```python
from build123d import *

# Parameters (mm, degrees)
SKETCH_1_W      = 35
SKETCH_1_H      = 80
EXTRUDE_1_DEPTH = 5
SKETCH_2_W      = 35
SKETCH_2_H      = 5
SKETCH_2_W_2    = 30
SKETCH_2_W_3    = 5
SKETCH_2_H_2    = 30
EXTRUDE_2_DEPTH = 45
FILLET_2_R      = 3


with BuildPart() as part:
    # 草圖1 → 填料-伸長1 (new body)
    with BuildSketch(Plane.XY):
        with Locations((-29.638177138, -5.194805195)):
            Rectangle(SKETCH_1_W, SKETCH_1_H)
    extrude(amount=EXTRUDE_1_DEPTH)

    # 草圖2 → 填料-伸長2 (add)
    with BuildSketch(Plane.XY.offset(5)):
        with Locations((-29.638177138, 32.305194805)):
            Rectangle(SKETCH_2_W, SKETCH_2_H)
        with Locations((-32.138177138, -42.694805195)):
            Rectangle(SKETCH_2_W_2, SKETCH_2_H)
        with Locations((-14.638177138, -42.694805195)):
            Rectangle(SKETCH_2_W_3, SKETCH_2_H)
        with Locations((-14.638177138, -25.194805195)):
            Rectangle(SKETCH_2_W_3, SKETCH_2_H_2)
    extrude(amount=EXTRUDE_2_DEPTH)

    # 圓角2
    fillet_2_edges = [part.edges().sort_by_distance(p)[0] for p in [
        (-47.138177138, -42.694805195, 50),
        (-14.638177138, -10.194805195, 50),
        (-47.138177138, 32.305194805, 50),
        (-12.138177138, 32.305194805, 50),
    ]]
    fillet(fillet_2_edges, radius=FILLET_2_R)


solid = part.part
```
Could you check a few things on this model? Use its own coordinates, in mm. A direction names the side the tool comes from. Round coordinates to 2 decimals unless told otherwise and drop trailing zeros. Loops run counter-clockwise (first coordinate to the right, second up) from the corner with the lowest first, then second, coordinate; pieces in that order, holes last. Notation, with made-up numbers: M -31,67 L 23,67 A8 ccw 23,82 Z; hole C 25.25,-17.75 d8. An arc over 180 degrees is marked long. Put each result on its own line as item: value.
Q1. For pin 1 (17.5 mm diameter, centred on x = -27.5, y = -9, fed in from +Z), with a flat end and sliding along its axis, tell me the tip position at first contact or that it passes through.
Check result:
pin 1: z = 5
Q2. Imagine slicing it at A-A (z = 20.5). Write out the boundary of the cut face in (x, y).
Check result:
outline: M -47.14,-45.19 L -12.14,-45.19 L -12.14,-10.19 L -17.14,-10.19 L -17.14,-40.19 L -47.14,-40.19 Z; M -47.14,29.81 L -12.14,29.81 L -12.14,34.81 L -47.14,34.81 Z
Q3. I need wall thicknesses on probe 1 along Y at (x, z) = (-28, 35); probe 2 along Y at (x, z) = (-13.5, 14.5); probe 3 along Z at (x, y) = (-33, 18.5). Which ranges of each line are inside material? Lowest first, please.
Check result:
probe 1: -45.19 to -40.19, 29.81 to 34.81
probe 2: -45.19 to -10.19, 29.81 to 34.81
probe 3: 0 to 5
Q4. Imagine slicing it at B-B (y = -24). Write out the boundary of the cut face in (x, z), then the cut area to 3 significant figures.
Check result:
outline: M -47.14,0 L -12.14,0 L -12.14,50 L -17.14,50 L -17.14,5 L -47.14,5 Z
area: 400 mm2
Q5. Imagine slicing it at D-D (y = -4.5). Write out the boundary of the cut face in (x, z), then the cut area to 3 significant figures.
Check result:
outline: M -47.14,0 L -12.14,0 L -12.14,5 L -47.14,5 Z
area: 175 mm2
Q6. Imagine slicing it at C-C (x = -18.5). Write out the boundary of the cut face in (y, z), then the cut area to 3 significant figures.
Check result:
outline: M -45.19,0 L 34.81,0 L 34.81,50 L 29.81,50 L 29.81,5 L -40.19,5 L -40.19,50 L -45.19,50 Z
area: 850 mm2
Q7. On a 3-axis mill with a long thin cutter (end or side, diameter ignored), from which of +Z, -Z, +X, -X, +Y, -Y can I reach the whole of each face in a straight line? I mean faces 5 (the face through (-17.138, -25, 27)), 6 (the face through (-46.28, -42.66, 49.1)), 7 (the face through (-30, 29.805, 27)), 8 (the face through (-12.994, 32.34, 49.098)), 9 (the face through (-30, -5, 0)). Say none if no direction works.
Check result:
face 5: +Z, -X
face 6: +Z, -X, +Y, -Y
face 7: +Z, +X, -X
face 8: +Z, +X, +Y
face 9: -Z, +X, -X, +Y, -Y
Q8. Thinking about a two-plate mould opening in Y: for faces 1 (the face through (-15, -10.195, 26)), 2 (the face through (-16, -35, 50)), 3 (the face through (-30, -45.195, 25)), 4 (the face through (-32, -40.195, 27)), which applies, released by +Y, released by -Y, zero draft, split by the parting line, or undercut?
Check result:
face 1: undercut
face 2: zero draft
face 3: released by -Y
face 4: undercut
